Drawing for the job (mm, zero at the part's lowest x, y, z). A direction names the side the tool comes from. Round coordinates to 2 decimals unless told otherwise and drop trailing zeros. Order: outer loops, then holes, each group sorted by start corner. A loop starts at its lowest first (then second) coordinate and runs counter-clockwise, first axis right, second up. Notation, with made-up numbers: M -19.75,-5.75 L -1.75,-5.75 A14 cw -1.75,18.25 Z; hole C -36,19 d7. An arc over 180 degrees is marked long. One line per item, written item: value. Start each with the question number.
Item 1: Two-plate mould, pull along X, no slides. Class the marked faces 1, 2 and 3: +X half, -X half, draft (parallel to the pull), parting line (faces both ways), or undercut.
Item 2: Band-saw the part on C-C, the plane y = 3.5. Write the cut outline in (x, z).
Item 3: Band-saw the part on D-D, the plane x = 9.5. Write the cut outline in (y, z), then the cut area to 3 significant figures.
Item 4: Probe L1, parallel to Y at x = 6, z = 7.5; L2, parallel to Z at x = 11.75, y = 6; L3, parallel to Y at x = 9.25, z = 7. List the from-to ranges inside material, lowest first.
Item 5: Band-saw the part on A-A, the plane z = 12.75. Write the cut outline in (x, y).
Item 6: Tool access for the marked faces 4, 5 and 6: list every direction of +Z, -Z, +X, -X, +Y, -Y with a clear straight run to the whole face (end or side of a thin tool).
Item 7: Pin check, flat tips, straight feed: pin 1 (1.1 mm diameter, centred on x = 3, y = 1.5, fed in from -Z); pin 2 (0.5 mm diameter, centred on y = 2.5, z = 4, fed in from +X); pin 3 (3.5 mm diameter, centred on x = 5.5, z = 12.5, fed in from +Y); pin 4 (5 mm diameter, centred on x = 6, y = 7, fed in from -Z). Stop position of each tip, or through.
Item 8: Band-saw the part on B-B, the plane y = 7. Write the cut outline in (x, z).
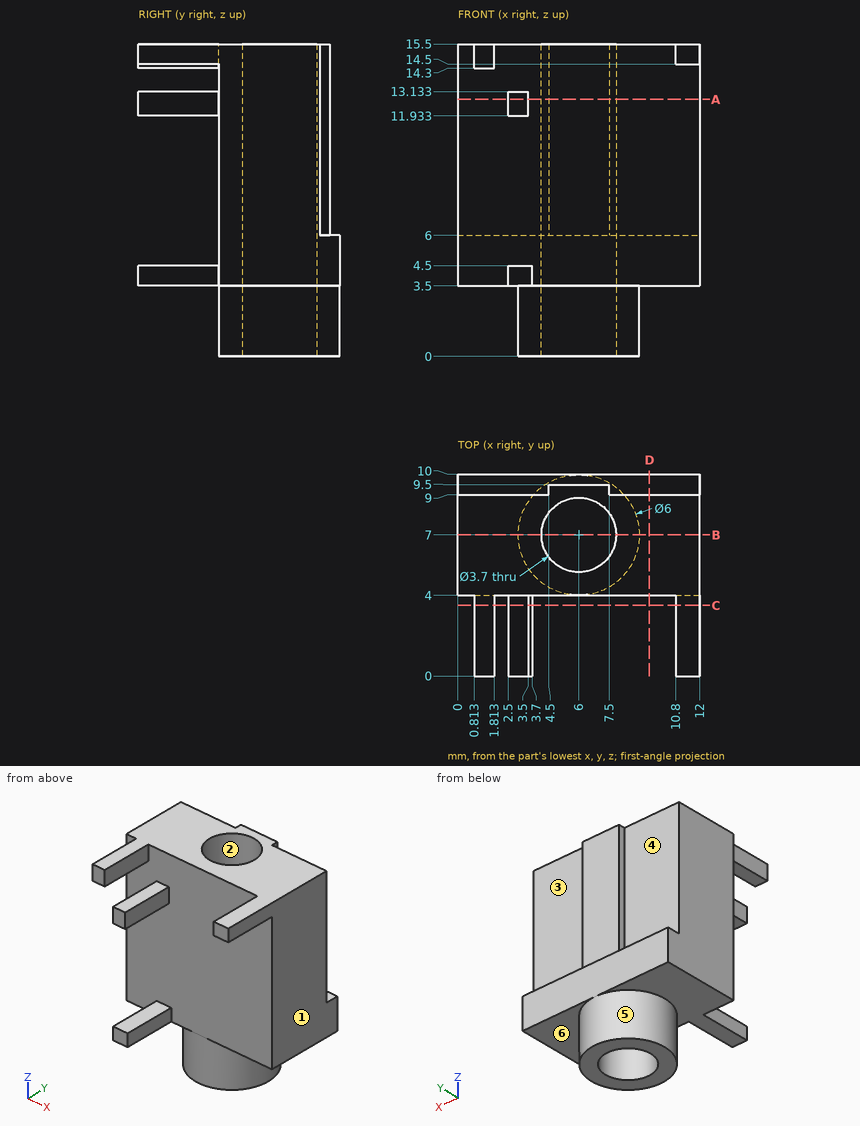
Output:
1. face 1: +X half
1. face 2: undercut
1. face 3: draft
2. outline: M 0.81,14.3 L 1.81,14.3 L 1.81,15.5 L 0.81,15.5 Z; M 2.5,3.5 L 3.7,3.5 L 3.7,4.5 L 2.5,4.5 Z; M 2.5,11.93 L 3.5,11.93 L 3.5,13.13 L 2.5,13.13 Z; M 10.8,14.5 L 12,14.5 L 12,15.5 L 10.8,15.5 Z
3. outline: M 4,3.5 L 10,3.5 L 10,6 L 9,6 L 9,15.5 L 4,15.5 Z
3. area: 62.5 mm²
4. L1: y = 4 to 5.15, 8.85 to 9.5
4. L2: z = 3.5 to 15.5
4. L3: y = 4 to 9
5. outline: M 0,4 L 2.5,4 L 2.5,0 L 3.5,0 L 3.5,4 L 12,4 L 12,9 L 7.5,9 L 7.5,9.5 L 4.5,9.5 L 4.5,9 L 0,9 Z; hole C 6,7 d3.7
6. face 4: +Z, -X, +Y
6. face 5: -Z
6. face 6: -Z, +X
7. pin 1: stops at z = 3.5
7. pin 2: stops at x = 3.7
7. pin 3: stops at y = 9.5
7. pin 4: stops at z = 0
8. outline: M 0,3.5 L 3,3.5 L 3,0 L 4.15,0 L 4.15,15.5 L 0,15.5 Z; M 7.85,0 L 9,0 L 9,3.5 L 12,3.5 L 12,15.5 L 7.85,15.5 Z
